Here's how the part is built. I have some questions about the finished solid (model axes, mm). A direction names the side the tool comes from. Round coordinates to 2 decimals unless told otherwise and drop trailing zeros. Write each loop counter-clockwise with the first axis right and the second up, starting at its lowest first coordinate (ties: lowest second). Pieces come first, ordered by that corner, then holes. Notation, with made-up numbers: (65.25, -25) - (104.25, -25) arc R27 ccw to (104.25, -7) - close; hole circle Ø4 at (78.25, 54.5). An arc over 180 degrees is marked (long way). Use one line per item in the form item = value. Start each with the question number.
1. Will these pins go through, and if not, where does the flat tip stop? pin 1 (1.8 mm diameter, centred on x = 23.5, y = -25.125, fed in from -Z); pin 2 (3.5 mm diameter, centred on x = -23.5, y = -25.125, fed in from -Z); pin 3 (10.5 mm diameter, centred on x = 8.5, z = 15, fed in from -Y) (3 decimals).
2. I want a section at D-D, the plane z = 11. List the corners of the cut face in (x, y) for me (1 decimal), plus the area to 3 significant figures.
3. Which directions (+Z, -Z, +X, -X, +Y, -Y) give clear straight access to the entire face, cutting with the end or side of a thin tool? Please do faces 5 (the flat face through (-7, 20, 0)), 6 (the cylindrical face through (-27.53, -29.124, -2.415)).
4. We'd pull the mould along X, two halves only. Please class faces 1 (the cylindrical face through (-24.606, 22.889, -2.348)), 2 (the cylindrical face through (-23.7, -23.64, -2.35)), 3 (the flat face through (-28.1, 10, -2)), 4 (the flat face through (0, 34.488, 10)): +X half, -X half, draft (parallel to the pull), parting line (faces both ways), or undercut.
5. I want a section at B-B, the plane x = 23.5. State how many separate pieces and enclosed holes the cut face has, plus the area to 3 significant figures.
6. If I drill on line 1 along Y through (x, z) = (23.5, -1.75) (3 decimals); line 2 along Y through (x, z) = (-23.5, -1.9) (3 decimals); line 3 along Y through (x, z) = (22.5, 1.5) (1 decimal), over which ranges is the centre line in solid material (lowest first)?
7. I want a section at C-C, the plane y = 14. List the corners of the cut face in (x, z) for me, plus the area to 3 significant figures.
```python
from build123d import *

# Parameters (mm, degrees)
SKETCH1_W                    = 56.2
SKETCH1_H                    = 59.45
SKETCH1_R                    = 20.52
SKETCH1_R_2                  = 1.5
BASE_FLANGE1_DEPTH           = 4.7625
EDGE_FLANGE1_STRIP_W         = 19.304
EDGE_FLANGE1_STRIP_H         = 4.7625
EDGE_FLANGE1_STRIP_CUT_DEPTH = 56.2
EDGE_FLANGE1_DEPTH           = 56.2
FILLET1_R                    = 2
CUT_EXTRUDE1_REACH           = 75.067
SKETCH11_R                   = 2


# Sheet-metal steps are written as plain solids
with BuildPart() as part:
    # Sketch1 → Base-Flange1 (new body)
    with BuildSketch(Plane.XY):
        Rectangle(SKETCH1_W, SKETCH1_H)
        Circle(SKETCH1_R, mode=Mode.SUBTRACT)
        with Locations((-23.5, 21.874999952)):
            Circle(SKETCH1_R_2, mode=Mode.SUBTRACT)
        with Locations((23.5, 21.874999952)):
            Circle(SKETCH1_R_2, mode=Mode.SUBTRACT)
        with Locations((-23.5, -25.125)):
            Circle(SKETCH1_R_2, mode=Mode.SUBTRACT)
        with Locations((23.5, -25.125)):
            Circle(SKETCH1_R_2, mode=Mode.SUBTRACT)
    extrude(amount=-BASE_FLANGE1_DEPTH)

    # Edge-Flange1 strip (across the edge) → Edge-Flange1 strip cut (cut)
    with BuildSketch(Plane(origin=(28.1, 29.725, 0), x_dir=(0, -1, 0), z_dir=(-1, 0, 0))):
        with Locations((-9.525, -2.38125)):
            Rectangle(EDGE_FLANGE1_STRIP_W, EDGE_FLANGE1_STRIP_H)
    extrude(amount=EDGE_FLANGE1_STRIP_CUT_DEPTH, mode=Mode.SUBTRACT)

    # Edge-Flange1 section (across the edge) → Edge-Flange1 (add)
    with BuildSketch(Plane(origin=(28.1, 29.725, 0), x_dir=(0, -1, 0), z_dir=(-1, 0, 0))):
        with BuildLine():
            Line((-4.7625, 0.127), (-4.7625, 20.6375))
            Line((-4.7625, 20.6375), (0, 20.6375))
            Line((0, 20.6375), (0, 0.127))
            ThreePointArc((0, 0.127), (0.037197439, 0.037197439), (0.127, 0))
            Line((0.127, 0), (0.127, -4.7625))
            ThreePointArc((0.127, -4.7625), (-3.330398607, -3.330398607), (-4.7625, 0.127))
        make_face()
    extrude(amount=EDGE_FLANGE1_DEPTH)

    # Fillet1
    fillet1_edges = [part.edges().sort_by_distance(p)[0] for p in [
        (28.1, 32.10625, 20.6375),
        (-28.1, 32.10625, 20.6375),
        (28.1, -29.725, -2.38125),
        (-28.1, -29.725, -2.38125),
    ]]
    fillet(fillet1_edges, radius=FILLET1_R)

    # Sketch11 → Cut-Extrude1 (cut, up to next)
    with BuildSketch(Plane(origin=(0, 34.4875, 0), x_dir=(1, 0, 0), z_dir=(0, 1, 0)), mode=Mode.PRIVATE) as cut_extrude1_sk1:
        with Locations(Location((-20, -10.7875, 0), (0, 0, 270))):
            Circle(SKETCH11_R)
    cut_extrude1_tool1 = extrude(cut_extrude1_sk1.sketch, amount=-CUT_EXTRUDE1_REACH, mode=Mode.PRIVATE) & part.part
    # Sketch11 → Cut-Extrude1 (cut, up to next)
    with BuildSketch(Plane(origin=(0, 34.4875, 0), x_dir=(1, 0, 0), z_dir=(0, 1, 0)), mode=Mode.PRIVATE) as cut_extrude1_sk2:
        with Locations(Location((20, -10.7875, 0), (0, 0, 270))):
            Circle(SKETCH11_R)
    cut_extrude1_tool2 = extrude(cut_extrude1_sk2.sketch, amount=-CUT_EXTRUDE1_REACH, mode=Mode.PRIVATE) & part.part
    add(cut_extrude1_tool1.solids().sort_by_distance((-20, 34.4875, 10.7875))[0], mode=Mode.SUBTRACT)
    add(cut_extrude1_tool2.solids().sort_by_distance((20, 34.4875, 10.7875))[0], mode=Mode.SUBTRACT)


solid = part.part
```
Model answer:
q1.pin_1 = through
q1.pin_2 = -4.76
q1.pin_3 = 29.725
q2.outline = (-28.1, 29.7) - (-22, 29.7) - (-22, 34.5) - (-28.1, 34.5) - close; (-18, 29.7) - (18, 29.7) - (18, 34.5) - (-18, 34.5) - close; (22, 29.7) - (28.1, 29.7) - (28.1, 34.5) - (22, 34.5) - close
q2.area = 230 mm2
q3.face_5 = +Z, +X, -X, -Y
q3.face_6 = +Z, -Z, -X, -Y
q4.face_1 = undercut
q4.face_2 = undercut
q4.face_3 = -X half
q4.face_4 = draft
q5.separate_pieces = 3
q5.enclosed_holes = 0
q5.area = 370 mm2
q6.line_1 = -29.725 to -26.625, -23.625 to 20.375, 23.375 to 34.113
q6.line_2 = -29.725 to -26.625, -23.625 to 20.375, 23.375 to 34.048
q6.line_3 = 29.7 to 34.5
q7.outline = (-28.1, -4.76) - (-15, -4.76) - (-15, 0) - (-28.1, 0) - close; (15, -4.76) - (28.1, -4.76) - (28.1, 0) - (15, 0) - close
q7.area = 125 mm2
